Work out the finished part from the listing and answer in its coordinate system (mm). A direction names the side the tool comes from. Coordinates: 2 decimals unless noted, no trailing zeros. Write each loop counter-clockwise with the first axis right and the second up, starting at its lowest first coordinate (ties: lowest second). Pieces come first, ordered by that corner, then holes. Notation, with made-up numbers: M 38,56.25 L 93,56.25 A21 cw 93,73.25 Z; hole C -38,-17.75 d8. An arc over 180 degrees is marked long. Answer as CSV lines item,"result". Start each with the question number.
(1) A cutting plane is placed at D-D on x = 25. Give the vertices of the cut face in (y, z), then the cut area to 3 significant figures.
(2) For faces 5 (the cylindrical face through (-29.97, 1.32, 29.58)), 6 (the flat face through (-2, 32, 60)), 7 (the cylindrical face through (15.925, -78.905, 106.975)), determine the directions among +Z, -Z, +X, -X, +Y, -Y from which every point of the face is accessible in a straight line to the end or side of a thin tool.
(3) The mould has two halves that part along Y. Classify faces 1 (the flat face through (-30, -36, 65)), 2 (the cylindrical face through (-2.153, -93.617, 132.325)), 3 (the flat face through (0, -105, 65)), 4 (the flat face through (0, -84, 120)): released by +Y, released by -Y, zero draft, split by the parting line, or undercut.
(4) A cutting plane is placed at C-C on z = 33.5. Give the vertices of the cut face in (x, y).
(5) Find the intervals of material crossed by L1, parallel to Y at x = 0, z = 139; L2, parallel to Z at x = 8.5, y = -25.5; L3, parallel to Z at x = 24.5, y = 25.5, in increasing order. Write a range as [from, to].
(6) Flat-ended cylindrical pins translate along their axes: P1, Ø4, axis at x = 16.5, y = -65.5, coming from the +Z side; P2, Ø3, axis at x = 18, z = 23.5, coming from the +Y side; P3, Ø4, axis at x = -4.5, z = 72.5, coming from the +Y side. Find the tip coordinate at first contact, or state that the pin passes through.
(7) A cutting plane is placed at A-A on x = 0. Give the vertices of the cut face in (y, z), then the cut area to 3 significant figures.
(8) A cutting plane is placed at B-B on y = -80. Give the vertices of the cut face in (x, z).
from build123d import *

# Parameters (mm, degrees)
F0_R     = 30
F1_DEPTH = 60
F2_W     = 60
F2_H     = 140
F3_DEPTH = 10
F4_R     = 16.695994
F5_DEPTH = 50
F6_R     = 16.695994
F6_R_2   = 9.933537
F7_DEPTH = 25


with BuildPart() as f1:
    # F0 (on Top) → F1 (new body)
    with BuildSketch(Plane.XY):
        Circle(F0_R)
    extrude(amount=F1_DEPTH)

    # F2 (on face) → F3 (join)
    with BuildSketch(Plane.XY.offset(60)):
        with Locations((0, -35)):
            Rectangle(F2_W, F2_H)
    extrude(amount=F3_DEPTH)

    # F4 (on face) → F5 (join)
    with BuildSketch(Plane.XY.offset(70)):
        with Locations((0, -83.919823)):
            Circle(F4_R)
    extrude(amount=F5_DEPTH)

    # F6 (on face) → F7 (join)
    with BuildSketch(Plane.XY.offset(120)):
        with Locations((0, -83.919823)):
            Circle(F6_R)
        with Locations((0, -83.919823)):
            Circle(F6_R_2, mode=Mode.SUBTRACT)
    extrude(amount=F7_DEPTH)


solid = f1.part
Here are the results:
1,outline,"M -105,60 L -16.58,60 L -16.58,0 L 16.58,0 L 16.58,60 L 35,60 L 35,70 L -105,70 Z"
1,area,"3,390 mm^2"
2,face 5,"-Z"
2,face 6,"-Z, +Y"
2,face 7,"+Z"
3,face 1,"zero draft"
3,face 2,"undercut"
3,face 3,"released by -Y"
3,face 4,"undercut"
4,outline,"C 0,0 d60"
5,L1,"y = [-100.62, -93.85], [-73.99, -67.22]"
5,L2,"z = [0, 70]"
5,L3,"z = [60, 70]"
6,P1,"stops at z = 70"
6,P2,"stops at y = 25.05"
6,P3,"stops at y = -67.41"
7,outline,"M -105,60 L -30,60 L -30,0 L 30,0 L 30,60 L 35,60 L 35,70 L -67.22,70 L -67.22,145 L -73.99,145 L -73.99,120 L -93.85,120 L -93.85,145 L -100.62,145 L -100.62,70 L -105,70 Z"
7,area,"7,010 mm^2"
8,outline,"M -30,60 L 30,60 L 30,70 L 16.23,70 L 16.23,145 L 9.13,145 L 9.13,120 L -9.13,120 L -9.13,145 L -16.23,145 L -16.23,70 L -30,70 Z"
